```python
from build123d import *

# Parameters (mm, degrees)
CROQUIS1_W                  = 41.8
CROQUIS1_H                  = 41.8
SALIENTE_EXTRUIR1_DEPTH     = 11.3
CROQUIS2_W                  = 42
CROQUIS2_H                  = 41.9
SALIENTE_EXTRUIR2_DEPTH     = 10.85
CROQUIS3_W                  = 10.85
CROQUIS3_H                  = 42
SALIENTE_EXTRUIR3_DEPTH     = 0.1
CROQUIS4_W                  = 42
CROQUIS4_H                  = 42
SALIENTE_EXTRUIR4_DEPTH     = 10.85
CORTAR_EXTRUIR1_REACH       = 26.9
CROQUIS5_W                  = 0.1
CROQUIS5_H                  = 28
CORTAR_EXTRUIR2_REACH       = 26.9
CROQUIS6_W                  = 28
CROQUIS6_H                  = 0.1
CROQUIS7_W                  = 2.75
CROQUIS7_H                  = 28
CORTAR_EXTRUIR3_DEPTH       = 0.1
CROQUIS8_W                  = 2.75
CROQUIS8_H                  = 28
CORTAR_EXTRUIR4_DEPTH       = 0.1
CROQUIS9_W                  = 28
CROQUIS9_H                  = 0.1
CORTAR_EXTRUIR5_DEPTH       = 2.75
CROQUIS10_W                 = 2.75
CROQUIS10_H                 = 28
CORTAR_EXTRUIR6_DEPTH       = 0.1
CROQUIS11_W                 = 2.75
CROQUIS11_H                 = 28
CORTAR_EXTRUIR7_DEPTH       = 0.1
CROQUIS12_W                 = 2.75
CROQUIS12_H                 = 28
CORTAR_EXTRUIR8_DEPTH       = 0.1
CHAFL_N1_SIZE               = 5.214213562
CHAFL_N2_SIZE               = 4
CROQUIS18_R                 = 2
CORTAR_EXTRUIR10_DEPTH      = 6
CORTAR_EXTRUIR10_DEPTH_BACK = 3


with BuildPart() as part:
    # Croquis1 → Saliente-Extruir1 (new body)
    with BuildSketch(Plane(origin=(-5.65, 0, 0), x_dir=(0, -1, 0), z_dir=(-1, 0, 0))):
        Rectangle(CROQUIS1_W, CROQUIS1_H)
    extrude(amount=-SALIENTE_EXTRUIR1_DEPTH)

    # Croquis2 → Saliente-Extruir2 (add)
    with BuildSketch(Plane(origin=(5.65, 0, 0), x_dir=(0, 0, -1), z_dir=(1, 0, 0))):
        with Locations((0, -0.05)):
            Rectangle(CROQUIS2_W, CROQUIS2_H)
    extrude(amount=SALIENTE_EXTRUIR2_DEPTH)

    # Croquis3 → Saliente-Extruir3 (add)
    with BuildSketch(Plane(origin=(0, 20.9, 0), x_dir=(-1, 0, 0), z_dir=(0, 1, 0))):
        with Locations((-11.075, 0)):
            Rectangle(CROQUIS3_W, CROQUIS3_H)
    extrude(amount=SALIENTE_EXTRUIR3_DEPTH)

    # Croquis4 → Saliente-Extruir4 (add)
    with BuildSketch(Plane(origin=(-5.65, 0, 0), x_dir=(0, 0, -1), z_dir=(1, 0, 0))):
        Rectangle(CROQUIS4_W, CROQUIS4_H)
    extrude(amount=-SALIENTE_EXTRUIR4_DEPTH)

    # Croquis5 → Cortar-Extruir1 (cut, up to next)
    with BuildSketch(Plane(origin=(8.4, 0, 0), x_dir=(0, 0, -1), z_dir=(1, 0, 0)), mode=Mode.PRIVATE) as cortar_extruir1_sk1:
        with Locations((20.95, 0)):
            Rectangle(CROQUIS5_W, CROQUIS5_H)
    cortar_extruir1_tool1 = extrude(cortar_extruir1_sk1.sketch, amount=-CORTAR_EXTRUIR1_REACH, mode=Mode.PRIVATE) & part.part
    add(cortar_extruir1_tool1.solids().sort_by_distance((8.4, 0, -20.95))[0], mode=Mode.SUBTRACT)

    # Croquis6 → Cortar-Extruir2 (cut, up to next)
    with BuildSketch(Plane(origin=(-8.4, 0, 0), x_dir=(0, -1, 0), z_dir=(-1, 0, 0)), mode=Mode.PRIVATE) as cortar_extruir2_sk1:
        with Locations((0, 20.95)):
            Rectangle(CROQUIS6_W, CROQUIS6_H)
    cortar_extruir2_tool1 = extrude(cortar_extruir2_sk1.sketch, amount=-CORTAR_EXTRUIR2_REACH, mode=Mode.PRIVATE) & part.part
    add(cortar_extruir2_tool1.solids().sort_by_distance((-8.4, 0, 20.95))[0], mode=Mode.SUBTRACT)

    # Croquis7 → Cortar-Extruir3 (cut)
    with BuildSketch(Plane.XZ.offset(21)):
        with Locations((7.025, 0)):
            Rectangle(CROQUIS7_W, CROQUIS7_H)
    extrude(amount=-CORTAR_EXTRUIR3_DEPTH, mode=Mode.SUBTRACT)

    # Croquis8 → Cortar-Extruir4 (cut)
    with BuildSketch(Plane.XY.offset(21)):
        with Locations((7.025, 0)):
            Rectangle(CROQUIS8_W, CROQUIS8_H)
    extrude(amount=-CORTAR_EXTRUIR4_DEPTH, mode=Mode.SUBTRACT)

    # Croquis9 → Cortar-Extruir5 (cut)
    with BuildSketch(Plane.ZY.offset(-5.65)):
        with Locations((0, 20.95)):
            Rectangle(CROQUIS9_W, CROQUIS9_H)
    extrude(amount=-CORTAR_EXTRUIR5_DEPTH, mode=Mode.SUBTRACT)

    # Croquis10 → Cortar-Extruir6 (cut)
    with BuildSketch(Plane.XZ.offset(21)):
        with Locations((-7.025, 0)):
            Rectangle(CROQUIS10_W, CROQUIS10_H)
    extrude(amount=-CORTAR_EXTRUIR6_DEPTH, mode=Mode.SUBTRACT)

    # Croquis11 → Cortar-Extruir7 (cut)
    with BuildSketch(Plane(origin=(0, 0, -21), x_dir=(-1, 0, 0), z_dir=(0, 0, -1))):
        with Locations((7.025, 0)):
            Rectangle(CROQUIS11_W, CROQUIS11_H)
    extrude(amount=-CORTAR_EXTRUIR7_DEPTH, mode=Mode.SUBTRACT)

    # Croquis12 → Cortar-Extruir8 (cut)
    with BuildSketch(Plane(origin=(0, 21, 0), x_dir=(-1, 0, 0), z_dir=(0, 1, 0))):
        with Locations((7.025, 0)):
            Rectangle(CROQUIS12_W, CROQUIS12_H)
    extrude(amount=-CORTAR_EXTRUIR8_DEPTH, mode=Mode.SUBTRACT)

    # Croquis15 → Revolución1 (revolve)
    with BuildSketch(Plane.XY):
        Polygon((15.5, 11), (15.5, 0), (33, 0), (33, 2.5), (18, 2.5), (18, 11), align=None)
    revolve(axis=Axis((15.5, 0, 0), (1, 0, 0)))

    # Chaflán1
    chafl_n1_edges = [part.edges().sort_by_distance(p)[0] for p in [
        (0, -20.9, -20.9),
        (0, 20.9, 20.9),
        (0, 20.9, -20.9),
        (0, -20.9, 20.9),
    ]]
    chamfer(chafl_n1_edges, length=CHAFL_N1_SIZE)

    # Chaflán2
    chafl_n2_edges = [part.edges().sort_by_distance(p)[0] for p in [
        (11.075, -21, 21),
        (11.075, -21, -21),
        (11.075, 21, 21),
        (11.075, 21, -21),
        (-11.075, 21, -21),
        (-11.075, -21, -21),
        (-11.075, -21, 21),
        (-11.075, 21, 21),
    ]]
    chamfer(chafl_n2_edges, length=CHAFL_N2_SIZE)

    # Croquis18 → Cortar-Extruir10 (cut, two sides)
    with BuildSketch(Plane(origin=(12.45, 0, 0), x_dir=(0, 0, -1), z_dir=(1, 0, 0))) as cortar_extruir10_sk:
        with Locations((-15.5, 15.5)):
            Circle(CROQUIS18_R)
        with Locations((15.5, 15.5)):
            Circle(CROQUIS18_R)
        with Locations((15.5, -15.5)):
            Circle(CROQUIS18_R)
        with Locations((-15.5, -15.5)):
            Circle(CROQUIS18_R)
    extrude(amount=CORTAR_EXTRUIR10_DEPTH, mode=Mode.SUBTRACT)
    extrude(cortar_extruir10_sk.sketch, amount=-CORTAR_EXTRUIR10_DEPTH_BACK, mode=Mode.SUBTRACT)


solid = part.part
```
The listing builds one solid part. Answer for the finished solid, in the listing's coordinates (mm). A direction names the side the tool comes from. Round coordinates to 2 decimals unless told otherwise and drop trailing zeros. Write each loop counter-clockwise with the first axis right and the second up, starting at its lowest first coordinate (ties: lowest second). Pieces come first, ordered by that corner, then holes. Notation, with made-up numbers: (51, 38.25) -> (64, 38.25) arc R30 ccw to (64, 73.25) -> close; hole circle Ø8 at (-25.75, -24.75). An arc over 180 degrees is marked (long way). Use CSV: the item, a comma, the result in double quotes. Start each with the question number.
(1) Section D-D on x = -1.5 is taken. Give the vertices of the cut face in (y, z).
(2) Section A-A on x = 15 is taken. Give the vertices of the cut face in (y, z), then the cut area to 3 significant figures.
(3) The mould has two halves that part along X. Classify faces 1 (the face through (-12, -21, 0)), 2 (the face through (-0.079, -18.329, -18.256)), 3 (the face through (-16.5, 0, 0)): released by +X, released by -X, zero draft, split by the parting line, or undercut.
(4) Section B-B on y = 0 is taken. Give the vertices of the cut face in (x, z).
(5) Consider L1, parallel to Y at x = 12, z = 15.5; L2, parallel to Z at x = 14, y = -15. Determine where each line is inside the solid, lowest interval first. Write a range as from..to.
(6) Each of these flat-tipped pins is pushed along its axis until it touches: pin 1 (1.5 mm diameter, centred on x = 27, z = -2, fed in from +Y); pin 2 (5 mm diameter, centred on x = 3.5, y = 7.5, fed in from +Z); pin 3 (12 mm diameter, centred on y = -3.5, z = -14.5, fed in from +X); pin 4 (1 mm diameter, centred on x = 19, z = 3.5, fed in from +Y). Where does it stop, or does it pass through?
(7) Which of the six approach directions +Z, -Z, +X, -X, +Y, -Y give full straight-line access (tool end or side, diameter ignored) to faces 4 (the face through (-11, 19, -19)), 5 (the face through (25.4, -0.54, -2.44)), 6 (the face through (-5.65, -18.5, -18.5)), 7 (the face through (5.65, 18.5, -18.6))?
A:
1,outline,"(-20.9, -15.69) -> (-15.69, -20.9) -> (15.69, -20.9) -> (20.9, -15.69) -> (20.9, 15.69) -> (15.69, 20.9) -> (-15.69, 20.9) -> (-20.9, 15.69) -> close"
2,outline,"(-21, -17) -> (-17, -21) -> (17, -21) -> (21, -17) -> (21, 17) -> (17, 21) -> (-17, 21) -> (-21, 17) -> close; hole circle Ø4 at (-15.5, -15.5); hole circle Ø4 at (-15.5, 15.5); hole circle Ø4 at (15.5, -15.5); hole circle Ø4 at (15.5, 15.5)"
2,area,"1,680 mm²"
3,face 1,"zero draft"
3,face 2,"undercut"
3,face 3,"released by -X"
4,outline,"(-16.5, -21) -> (-8.4, -21) -> (-8.4, -20.9) -> (8.4, -20.9) -> (8.4, -21) -> (16.5, -21) -> (16.5, -11) -> (18, -11) -> (18, -2.5) -> (33, -2.5) -> (33, 2.5) -> (18, 2.5) -> (18, 11) -> (16.5, 11) -> (16.5, 21) -> (8.4, 21) -> (8.4, 20.9) -> (-8.4, 20.9) -> (-8.4, 21) -> (-16.5, 21) -> close"
5,L1,"y = -21..-17.5, -13.5..13.5, 17.5..21"
5,L2,"z = -21..-17.44, -13.56..13.56, 17.44..21"
6,pin 1,"stops at y = 2.17"
6,pin 2,"stops at z = 20.9"
6,pin 3,"stops at x = 18"
6,pin 4,"passes through"
7,face 4,"-Z, +X, -X, +Y"
7,face 5,"+X"
7,face 6,"-Z, -Y"
7,face 7,"-Z, +Y"
